```python
from build123d import *

# Parameters (mm, degrees)
F0_R     = 4.1
F1_DEPTH = 13
F2_R     = 1.327998
F2_R_2   = 1.395389
F3_DEPTH = 15


with BuildPart() as f1:
    # F0 (on Front) → F1 (new body)
    with BuildSketch(Plane.XZ):
        with BuildLine():
            Line((-36.756809, 10.154071), (-36.988087, 0.408211))
            ThreePointArc((-36.988087, 0.408211), (-31.234461, -6.890291), (-23.304849, -2.043272))
            Line((-23.304849, -2.043272), (-21.400974, 7.909327))
            ThreePointArc((-21.400974, 7.909327), (-20.366079, 9.657697), (-18.454402, 10.345665))
            Line((-18.454402, 10.345665), (-9.227201, 10.345665))
            Line((-9.227201, 10.345665), (0, 10.345665))
            Line((0, 10.345665), (10, 10.345665))
            Line((10, 10.345665), (20, 10.345665))
            ThreePointArc((20, 10.345665), (22.12132, 9.466985), (23, 7.345665))
            Line((23, 7.345665), (23, 0))
            ThreePointArc((23, 0), (30, -7), (37, 0))
            Line((37, 0), (37, 9.456913))
            ThreePointArc((37, 9.456913), (35.535534, 12.992447), (32, 14.456913))
            Line((32, 14.456913), (1.21127, 14.456913))
            Line((1.21127, 14.456913), (-1.21127, 14.456913))
            Line((-1.21127, 14.456913), (-31.805651, 14.456913))
            ThreePointArc((-31.805651, 14.456913), (-35.085453, 13.230889), (-36.756809, 10.154071))
        make_face()
        with Locations((-30, 0)):
            Circle(F0_R, mode=Mode.SUBTRACT)
        with Locations((30, 0)):
            Circle(F0_R, mode=Mode.SUBTRACT)
    extrude(amount=F1_DEPTH)

    # F2 (on face) → F3 (cut)
    with BuildSketch(Plane.XY.offset(14.456913)):
        with Locations((-20, -9.715236)):
            Circle(F2_R)
        with Locations((32.1, -4.615236)):
            Circle(F2_R_2)
    extrude(amount=-F3_DEPTH, mode=Mode.SUBTRACT)


solid = f1.part
```
CAD build for the part. Positions are in the model's coordinates, mm. A direction names the side the tool comes from. Round coordinates to 2 decimals unless told otherwise and drop trailing zeros. Order: outer loops, then holes, each group sorted by start corner. A loop starts at its lowest first (then second) coordinate and runs counter-clockwise, first axis right, second up.
Item 1: Tool access for faces 1 (the face through (33.431, -4.196, 8.386)), 2 (the face through (-34.096, -6.409, 0.18)), 3 (the face through (23, -6, 4)): list every direction of +Z, -Z, +X, -X, +Y, -Y with a clear straight run to the whole face (end or side of a thin tool).
Item 2: Saw through at A-A on x = -30. Write the cut outline in (y, z), then the cut area to 3 significant figures.
Item 3: Probe line 1 along Y through (x, z) = (32.1, 7); line 2 along Z through (x, y) = (30, -5.5); line 3 along Y through (x, z) = (-20, 10.75). List the from-to ranges inside material, lowest first.
Item 4: Pin check, flat tips, straight feed: pin 1 (6 mm diameter, centred on y = -5.5, z = 3.5, fed in from -X); pin 2 (1 mm diameter, centred on y = -10, z = 3.5, fed in from -X); pin 3 (2 mm diameter, centred on x = 10, y = -3.5, fed in from -Z). Stop position of each tip, or through.
Item 5: Mould opens along Y. For faces 4 (the face through (-35.05, -6.41, 13.26)), 5 (the face through (-21.327, -9.657, 12.069)), 6 (the face through (-1, 0, 11)) say: pulls with the +Y half, pulls with the -Y half, needs draft (parallel to the pull), parting line crosses it, or undercut.
Item 6: Saw through at D-D on z = 13.25. Write the cut outline in (x, y).
Item 7: Saw through at B-B on z = -5. Write the cut outline in (x, y).
Item 8: Saw through at C-C on y = -7. Write the cut outline in (x, z), then the cut area to 3 significant figures.
Reported:
1. face 1: +Z
1. face 2: +Y, -Y
1. face 3: -Z, +Y, -Y
2. outline: (-13, -7) - (0, -7) - (0, -4.1) - (-13, -4.1) - close; (-13, 4.1) - (0, 4.1) - (0, 14.46) - (-13, 14.46) - close
2. area: 172 mm2
3. line 1: y = -13 to -6.01, -3.22 to 0
3. line 2: z = -7 to -4.1, 4.1 to 14.46
3. line 3: y = -13 to -11.04, -8.39 to 0
4. pin 1: stops at x = -36.99
4. pin 2: stops at x = -36.93
4. pin 3: stops at z = 10.35
5. face 4: needs draft
5. face 5: undercut
5. face 6: pulls with the +Y half
6. outline: (-35.06, -13) - (35.26, -13) - (35.26, 0) - (-35.06, 0) - close; hole circle Ø2.66 at (-20, -9.72); hole circle Ø2.79 at (32.1, -4.62)
7. outline: (-34.9, -13) - (-25.1, -13) - (-25.1, 0) - (-34.9, 0) - close; (25.1, -13) - (34.9, -13) - (34.9, 0) - (25.1, 0) - close
8. outline: (-36.99, 0.41) arc R7 ccw to (-23.3, -2.04) - (-21.4, 7.91) arc R3 cw to (-18.45, 10.35) - (20, 10.35) arc R3 cw to (23, 7.35) - (23, 0) arc R7 ccw to (37, 0) - (37, 9.46) arc R5 ccw to (32, 14.46) - (-31.81, 14.46) arc R5 ccw to (-36.76, 10.15) - close; hole circle Ø8.2 at (-30, 0); hole circle Ø8.2 at (30, 0)
8. area: 644 mm2
